Geometry: final body of the model. Coordinates: model frame, mm. A direction names the side the tool comes from. Round coordinates to 2 decimals unless told otherwise and drop trailing zeros. Loops run counter-clockwise (first coordinate to the right, second up) from the corner with the lowest first, then second, coordinate; pieces in that order, holes last. Notation, with made-up numbers: (40.25, 19.5) -> (92.25, 19.5) arc R30 ccw to (92.25, 41.5) -> close; hole circle Ø8 at (20, 85.5). An arc over 180 degrees is marked (long way). Answer in a Markdown table with one row per item.
```python
from build123d import *

# Parameters (mm, degrees)
SKETCH1_W               = 139.7
SKETCH1_H               = 76.2
SKETCH1_W_2             = 133.35
SKETCH1_H_2             = 69.85
BOSS_EXTRUDE1_DEPTH     = 228.6
SKETCH2_R               = 4
CUT_EXTRUDE1_DEPTH      = 271.602402059
CUT_EXTRUDE2_DEPTH      = 251.885277567
CUT_EXTRUDE2_DEPTH_BACK = 251.885277567


with BuildPart() as part:
    # Sketch1 → Boss-Extrude1 (new body)
    with BuildSketch(Plane(origin=(0, 0, 0), x_dir=(1, 0, 0), z_dir=(0, 1, 0))):
        Rectangle(SKETCH1_W, SKETCH1_H)
        Rectangle(SKETCH1_W_2, SKETCH1_H_2, mode=Mode.SUBTRACT)
    extrude(amount=BOSS_EXTRUDE1_DEPTH)

    # Sketch2 → Cut-Extrude1 (cut, through all)
    with BuildSketch(Plane(origin=(69.85, 0, 0), x_dir=(0, 0, -1), z_dir=(1, 0, 0))):
        with Locations((0, 209.55)):
            Circle(SKETCH2_R)
        with BuildLine():
            Line((-38.1, 203.2), (-38.1, 228.6))
            Line((-38.1, 228.6), (-12.7, 228.6))
            ThreePointArc((-12.7, 228.6), (-30.660512242, 221.160512242), (-38.1, 203.2))
        make_face()
        with BuildLine():
            Line((12.7, 228.6), (38.1, 228.6))
            Line((38.1, 228.6), (38.1, 203.2))
            ThreePointArc((38.1, 203.2), (30.660512242, 221.160512242), (12.7, 228.6))
        make_face()
    extrude(amount=-CUT_EXTRUDE1_DEPTH, mode=Mode.SUBTRACT)

    # Sketch3 → Cut-Extrude2 (cut, two sides: drawn at the far end of the back side and taken through both)
    with BuildSketch(Plane.XY.offset(38.1).offset(-CUT_EXTRUDE2_DEPTH_BACK)):
        with BuildLine():
            Line((-57.15, 82.55), (-57.15, 228.6))
            Line((-57.15, 228.6), (57.15, 228.6))
            Line((57.15, 228.6), (57.15, 82.55))
            ThreePointArc((57.15, 82.55), (0, 25.4), (-57.15, 82.55))
        make_face()
    extrude(amount=CUT_EXTRUDE2_DEPTH + CUT_EXTRUDE2_DEPTH_BACK, mode=Mode.SUBTRACT)


solid = part.part
```
Item 1: Line query: probe 1 along X at (y, z) = (34, 17.5) (3 decimals); probe 2 along Y at (x, z) = (67, 0); probe 3 along Z at (x, y) = (47.5, 46) (3 decimals). Output: solid intervals per line, ascending. Write a range as [from, to].
Answer:
| item | result |
|---|---|
| probe 1 | x = [-69.85, -66.675], [66.675, 69.85] |
| probe 2 | y = [0, 205.55], [213.55, 228.6] |
| probe 3 | z = [-38.1, -34.925], [34.925, 38.1] |
Item 2: Cut plane A-A (x = 0). Output: boundary loops of the cut face in (y, z) (3 decimals), then the cut area to 3 significant figures.
Answer:
| item | result |
|---|---|
| outline | (0, -38.1) -> (25.4, -38.1) -> (25.4, -34.925) -> (0, -34.925) -> close; (0, 34.925) -> (25.4, 34.925) -> (25.4, 38.1) -> (0, 38.1) -> close |
| area | 161 mm² |
Item 3: Cut plane B-B (z = 0). Output: boundary loops of the cut face in (x, y) (3 decimals).
Answer:
| item | result |
|---|---|
| outline | (-69.85, 0) -> (-66.675, 0) -> (-66.675, 205.55) -> (-69.85, 205.55) -> close; (-69.85, 213.55) -> (-66.675, 213.55) -> (-66.675, 228.6) -> (-69.85, 228.6) -> close; (66.675, 0) -> (69.85, 0) -> (69.85, 205.55) -> (66.675, 205.55) -> close; (66.675, 213.55) -> (69.85, 213.55) -> (69.85, 228.6) -> (66.675, 228.6) -> close |
Item 4: Draft query along Z for faces 1 (the face through (65, 213.681, -35.837)), 2 (the face through (69.85, 113, 1)), 3 (the face through (-25, 27, 34.925)), 4 (the face through (65, 214.19, 35.6)). Return one class per face: pulls with the +Z half, pulls with the -Z half, needs draft (parallel to the pull), parting line crosses it, or undercut.
Answer:
| item | result |
|---|---|
| face 1 | pulls with the -Z half |
| face 2 | needs draft |
| face 3 | undercut |
| face 4 | pulls with the +Z half |
Item 5: Cut plane C-C (y = 178.5). Output: boundary loops of the cut face in (x, z) (3 decimals), then the cut area to 3 significant figures.
Answer:
| item | result |
|---|---|
| outline | (-69.85, -38.1) -> (-57.15, -38.1) -> (-57.15, -34.925) -> (-66.675, -34.925) -> (-66.675, 34.925) -> (-57.15, 34.925) -> (-57.15, 38.1) -> (-69.85, 38.1) -> close; (57.15, -38.1) -> (69.85, -38.1) -> (69.85, 38.1) -> (57.15, 38.1) -> (57.15, 34.925) -> (66.675, 34.925) -> (66.675, -34.925) -> (57.15, -34.925) -> close |
| area | 605 mm² |
Item 6: Cut plane D-D (z = 30). Output: boundary loops of the cut face in (x, y) (3 decimals), then the cut area to 3 significant figures.
Answer:
| item | result |
|---|---|
| outline | (-69.85, 0) -> (-66.675, 0) -> (-66.675, 221.798) -> (-69.85, 221.798) -> close; (66.675, 0) -> (69.85, 0) -> (69.85, 221.798) -> (66.675, 221.798) -> close |
| area | 1,410 mm² |
Item 7: Reachability of faces 5 (the face through (-69.85, 113, 1)), 6 (the face through (-66.675, 113, 0)) from +Z, -Z, +X, -X, +Y, -Y: full face, straight path, thin tool, end or side. Return the list, or none.
Answer:
| item | result |
|---|---|
| face 5 | +Z, -Z, -X, +Y, -Y |
| face 6 | +Y, -Y |
Item 8: Pin query (flat end, axial travel): pin 1 Ø13 at (y, z) = (209.55, 0) entering from +X. Return the tip coordinate at first contact, or that it passes through.
Answer:
| item | result |
|---|---|
| pin 1 | stops at x = 69.85 |
